Source: CAD feature listing. Evaluate the final solid. Frame: model axes, mm. Face numbers are marked on the shaded views. A direction names the side the tool comes from. Give positions to 0.01 mm unless a question says otherwise; leave off trailing zeros. Order: outer loops, then holes, each group sorted by start corner. A loop starts at its lowest first (then second) coordinate and runs counter-clockwise, first axis right, second up.
1) Section B-B, the plane x = 43. Return loops of the section in (y, z), plus the area to 3 significant figures.
2) First-contact query: P1, Ø1.2, axis at x = 19.5, z = 0.5, coming from the -Y side; P2, Ø4, axis at x = 62.05, y = -70.64, coming from the +Z side; P3, Ø3, axis at x = 62.05, y = -70.64, coming from the +Z side; P4, Ø3, axis at y = -92.5, z = 2, coming from the -X side. Flat tips, straight axial feed; report the tip coordinate or a pass-through.
3) Access query for the marked faces 1 and 2. Directions: +Z, -Z, +X, -X, +Y, -Y. A direction counts if a zero-diameter tool reaches every point of the face in a straight line with its end or side. Return the directions, or none.
4) Material intervals for line 1 (Y direction, x = 60, z = 1.2); line 2 (X direction, y = -91, z = 3.55); line 3 (Y direction, x = 52, z = 3.4), sorted ascending.
5) Section A-A, the plane y = -84. Return loops of the section in (x, z), plus the area to 3 significant figures.
```python
from build123d import *

# Parameters (mm, degrees)
SKETCH1_R                                    = 1.25
SKETCH1_W                                    = 36
SKETCH1_H                                    = 42.1
BOSS_EXTRUDE1_DEPTH                          = 5
CSK_FOR_M3_COUNTERSUNK_FLAT_HEAD_SCR_2_COUNT = 2
CSK_FOR_M3_COUNTERSUNK_FLAT_HEAD_SCR_2_PITCH = 48.1
CSK_FOR_M3_COUNTERSUNK_FLAT_HEAD_SCR_3_COUNT = 2
CSK_FOR_M3_COUNTERSUNK_FLAT_HEAD_SCR_3_PITCH = 63.856166499
CSK_FOR_M3_COUNTERSUNK_FLAT_HEAD_SCR_4_COUNT = 2
CSK_FOR_M3_COUNTERSUNK_FLAT_HEAD_SCR_4_PITCH = 42
FURO_COM_FOLGA_DE_M34_D                      = 2.87
FILETE1_R                                    = 3
ESBO_O3_W                                    = 1.5
ESBO_O3_H                                    = 2.87
CORTE_EXTRUS_O1_DEPTH                        = 63
CORTE_EXTRUS_O1_DEPTH_BACK                   = 10


with BuildPart() as part:
    # Sketch1 → Boss-Extrude1 (new body)
    with BuildSketch(Plane.XY):
        with BuildLine():
            Line((20.053938932, -66.638943184), (63.053938932, -66.638943184))
            ThreePointArc((63.053938932, -66.638943184), (65.175259276, -67.517622841), (66.053938932, -69.638943184))
            Line((66.053938932, -69.638943184), (66.053938932, -119.738943184))
            ThreePointArc((66.053938932, -119.738943184), (65.175259276, -121.860263528), (63.053938932, -122.738943184))
            Line((63.053938932, -122.738943184), (20.053938932, -122.738943184))
            ThreePointArc((20.053938932, -122.738943184), (16.310928808, -120.149572552), (17.413938931, -115.73388079))
            Line((17.413938931, -115.73388079), (17.413938931, -73.644005579))
            ThreePointArc((17.413938931, -73.644005579), (16.310928808, -69.228313817), (20.053938932, -66.638943184))
        make_face()
        with Locations((20.053938932, -70.638943184)):
            Circle(SKETCH1_R, mode=Mode.SUBTRACT)
        with Locations((20.053938932, -118.738943184)):
            Circle(SKETCH1_R, mode=Mode.SUBTRACT)
        with Locations((62.053938932, -70.638943184)):
            Circle(SKETCH1_R, mode=Mode.SUBTRACT)
        with Locations((62.053938932, -118.738943184)):
            Circle(SKETCH1_R, mode=Mode.SUBTRACT)
        with Locations((41.053938932, -94.688943184)):
            Rectangle(SKETCH1_W, SKETCH1_H, mode=Mode.SUBTRACT)
    extrude(amount=BOSS_EXTRUDE1_DEPTH)

    # Sketch2 → CSK for M3 Countersunk Flat Head Screw1 (revolve, cut)
    with BuildSketch(Plane(origin=(20.053938932, -118.738943184, 5), x_dir=(0, -1, 0), z_dir=(1, 0, 0))):
        Polygon((0, 0), (0, 5), (1.6, 5), (1.6, 2.05), (3.15, 0.5), (3.15, 0), align=None)
    csk_for_m3_countersunk_flat_head_screw1 = revolve(axis=Axis((20.053938932, -118.738943184, 11.35), (0, 0, -1)), mode=Mode.SUBTRACT)

    # CSK for M3 Countersunk Flat Head Scr 2: CSK for M3 Countersunk Flat Head Screw1 ×2
    with Locations(*[(0, i * CSK_FOR_M3_COUNTERSUNK_FLAT_HEAD_SCR_2_PITCH, 0) for i in range(1, CSK_FOR_M3_COUNTERSUNK_FLAT_HEAD_SCR_2_COUNT)]):
        add(csk_for_m3_countersunk_flat_head_screw1, mode=Mode.SUBTRACT)

    # CSK for M3 Countersunk Flat Head Scr 3: CSK for M3 Countersunk Flat Head Screw1 ×2
    with Locations(*[Vector(0.657728177, 0.753255365, 0) * (i * CSK_FOR_M3_COUNTERSUNK_FLAT_HEAD_SCR_3_PITCH) for i in range(1, CSK_FOR_M3_COUNTERSUNK_FLAT_HEAD_SCR_3_COUNT)]):
        add(csk_for_m3_countersunk_flat_head_screw1, mode=Mode.SUBTRACT)

    # CSK for M3 Countersunk Flat Head Scr 4: CSK for M3 Countersunk Flat Head Screw1 ×2
    with Locations(*[(i * CSK_FOR_M3_COUNTERSUNK_FLAT_HEAD_SCR_4_PITCH, 0, 0) for i in range(1, CSK_FOR_M3_COUNTERSUNK_FLAT_HEAD_SCR_4_COUNT)]):
        add(csk_for_m3_countersunk_flat_head_screw1, mode=Mode.SUBTRACT)

    # Furo com folga de M34 (through all)
    with Locations(Plane(origin=(66.053938932, 0, 0), x_dir=(0, 0, -1), z_dir=(1, 0, 0))):
        with Locations((-1.5, -79.188943184), (-1.5, -110.188943184)):
            Hole(FURO_COM_FOLGA_DE_M34_D / 2)

    # Filete1
    filete1_edges = [part.edges().sort_by_distance(p)[0] for p in [
        (17.413938931, -115.73388079, 2.5),
        (17.413938931, -73.644005579, 2.5),
    ]]
    fillet(filete1_edges, radius=FILETE1_R)

    # Esboço3 → Corte-extrusão1 (cut, two sides)
    with BuildSketch(Plane.ZY.offset(-59.053938932)) as corte_extrus_o1_sk:
        with Locations((0.75, -79.188943184)):
            Rectangle(ESBO_O3_W, ESBO_O3_H)
        with Locations((0.75, -110.188943184)):
            Rectangle(ESBO_O3_W, ESBO_O3_H)
    extrude(amount=CORTE_EXTRUS_O1_DEPTH, mode=Mode.SUBTRACT)
    extrude(corte_extrus_o1_sk.sketch, amount=-CORTE_EXTRUS_O1_DEPTH_BACK, mode=Mode.SUBTRACT)


solid = part.part
```
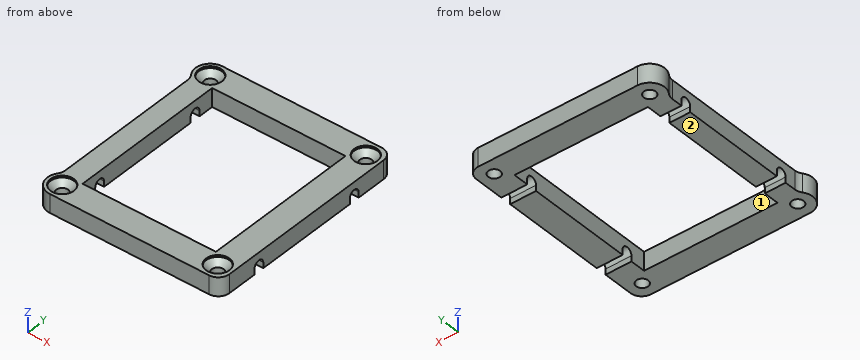
From the geometry:
1. outline: (-122.74, 0) - (-115.74, 0) - (-115.74, 5) - (-122.74, 5) - close; (-73.64, 0) - (-66.64, 0) - (-66.64, 5) - (-73.64, 5) - close
1. area: 70.0 mm2
2. P1: stops at y = -122.74
2. P2: stops at z = 3.35
2. P3: passes through
2. P4: stops at x = 17.41
3. face 1: +Z, -Z
3. face 2: -Z, +X, -X, +Y, -Y
4. line 1: y = -122.74 to -111.62, -108.75 to -80.62, -77.75 to -66.64
4. line 2: x = 17.41 to 23.05, 59.05 to 66.05
4. line 3: y = -122.74 to -115.74, -73.64 to -66.64
5. outline: (17.41, 0) - (23.05, 0) - (23.05, 5) - (17.41, 5) - close; (59.05, 0) - (66.05, 0) - (66.05, 5) - (59.05, 5) - close
5. area: 63.2 mm2
